Work out the finished part from the listing and answer in its coordinate system (mm). Face numbers are marked on the shaded views. Coordinates: 2 decimals unless noted, no trailing zeros. Order: outer loops, then holes, each group sorted by start corner. A loop starts at its lowest first (then second) coordinate and runs counter-clockwise, first axis right, second up.
1. The part is cut by section B-B, the plane y = -35. Give the vertices of the cut face in (x, z), then the cut area to 3 significant figures.
2. Flat-ended cylindrical pins translate along their axes: pin 1 Ø3.5 at (x, z) = (-9.5, -24) entering from -Y; pin 2 Ø11 at (x, y) = (-1, -16) entering from +Z; pin 3 Ø5 at (x, y) = (2, -10.5) entering from -Z; pin 4 Ø6 at (x, z) = (14.5, 92.5) entering from +Y. Find the tip coordinate at first contact, or state that the pin passes through.
3. Determine the mould class of the marked faces 1, 2, 3 and 4 for opening direction X: +X half, -X half, draft (parallel to the pull), parting line (faces both ways), or undercut.
4. Find the intervals of material crossed by probe 1 along Z at (x, y) = (-9.5, -3.25); probe 2 along Y at (x, z) = (11, -19); probe 3 along X at (y, z) = (-69, 92), in increasing order.
5. The part is cut by section C-C, the plane x = 18. Give the vertices of the cut face in (y, z).
6. The part is cut by section A-A, the plane z = 90.5. Give the vertices of the cut face in (x, y).
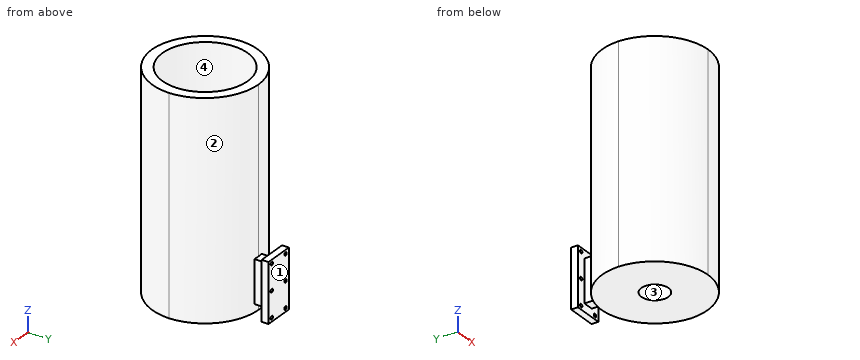
```python
from build123d import *

# Parameters (mm, degrees)
F0_W          = 28
F0_H          = 55
F0_R          = 1.6
F1_DEPTH      = 6.35
F2_W          = 10
F2_H          = 40
F3_DEPTH      = 12.7
F4_W          = 100
F4_H          = 200
F5_DEPTH      = 100
F6_R          = 40
F7_DEPTH      = 177.8
F8_R          = 12.7
F9_DEPTH      = 41.656
F10_T1_DEPTH  = 454
F10_T6_DEPTH  = 454
F10_T12_DEPTH = 454
F10_T18_DEPTH = 454
F10_T25_DEPTH = 454
F10_T31_DEPTH = 454
F10_T37_DEPTH = 454
F10_T43_DEPTH = 454
F10_T49_DEPTH = 454
F10_T56_DEPTH = 454
F10_T62_DEPTH = 454


# Not quite as in the source:
# - a fillet or chamfer that OpenCascade refuses, or shapes differently, is made with other operations: its cross-section is extruded or revolved along the edge and cut away or added


with BuildPart() as f1:
    # F0 (on Front) → F1 (new body)
    with BuildSketch(Plane.XZ):
        Rectangle(F0_W, F0_H)
        with Locations((-9.5, -24)):
            Circle(F0_R, mode=Mode.SUBTRACT)
        with Locations((9.5, -24)):
            Circle(F0_R, mode=Mode.SUBTRACT)
        with Locations((-9.5, 0)):
            Circle(F0_R, mode=Mode.SUBTRACT)
        with Locations((-9.5, 24)):
            Circle(F0_R, mode=Mode.SUBTRACT)
        with Locations((9.5, 0)):
            Circle(F0_R, mode=Mode.SUBTRACT)
        with Locations((9.5, 24)):
            Circle(F0_R, mode=Mode.SUBTRACT)
    extrude(amount=F1_DEPTH)

    # F2 (on face) → F3 (join)
    with BuildSketch(Plane.XZ.offset(6.35)):
        Rectangle(F2_W, F2_H)
    extrude(amount=F3_DEPTH)

    # F4 (on face) → F5 (join)
    with BuildSketch(Plane.XZ.offset(19.05)):
        with Locations((0, 72.5)):
            Rectangle(F4_W, F4_H)
    extrude(amount=F5_DEPTH)

    # F6 (on face) → F7 (cut)
    with BuildSketch(Plane.XY.offset(172.5)):
        with Locations((0, -69.05)):
            Circle(F6_R)
    extrude(amount=-F7_DEPTH, mode=Mode.SUBTRACT)

    # F8 (on face) → F9 (cut)
    with BuildSketch(Plane.XY.offset(-5.3)):
        with Locations((0, -69.05)):
            Circle(F8_R)
    extrude(amount=-F9_DEPTH, mode=Mode.SUBTRACT)

    # F10: fillet of radius 50.8 on 4 edges, made by hand

    # F10_s2 → F10_t1 (cut)
    with BuildSketch(Plane.XY.offset(-154.5)):
        with BuildLine():
            ThreePointArc((-0.8, -119.05), (35.1210244843, -104.1710244843), (50, -68.25))
            Line((50, -68.25), (50, -119.05))
            Line((50, -119.05), (-0.8, -119.05))
        make_face()
        with BuildLine():
            ThreePointArc((-50, -68.25), (-35.1210244843, -104.1710244843), (0.8, -119.05))
            Line((0.8, -119.05), (-50, -119.05))
            Line((-50, -119.05), (-50, -68.25))
        make_face()
    extrude(amount=F10_T1_DEPTH, mode=Mode.SUBTRACT)


with BuildPart() as f10_tool4:
    # F10_s5 → F10_t6 (new body)
    with BuildSketch(Plane.XY.offset(-154.5)):
        with BuildLine():
            ThreePointArc((-0.8, -19.05), (35.1210244843, -33.9289755157), (50, -69.85))
            Line((50, -69.85), (50, -19.05))
            Line((50, -19.05), (-0.8, -19.05))
        make_face()
    extrude(amount=F10_T6_DEPTH)

    split(bisect_by=Plane.XY.offset(-20), keep=Keep.BOTTOM)

    split(bisect_by=Plane.YZ.offset(5), keep=Keep.BOTTOM)


with BuildPart() as f1_1:
    add(f1.part)

    # F10_t3: cut F10_tool4
    add(f10_tool4.part, mode=Mode.SUBTRACT)


with BuildPart() as f10_tool10:
    # F10_s11 → F10_t12 (new body)
    with BuildSketch(Plane.XY.offset(-154.5)):
        with BuildLine():
            ThreePointArc((-0.8, -19.05), (35.1210244843, -33.9289755157), (50, -69.85))
            Line((50, -69.85), (50, -19.05))
            Line((50, -19.05), (-0.8, -19.05))
        make_face()
    extrude(amount=F10_T12_DEPTH)

    split(bisect_by=Plane.XY.offset(-20), keep=Keep.BOTTOM)

    split(bisect_by=Plane.YZ.offset(5), keep=Keep.TOP)


with BuildPart() as f1_2:
    add(f1_1.part)

    # F10_t9: cut F10_tool10
    add(f10_tool10.part, mode=Mode.SUBTRACT)


with BuildPart() as f10_tool16:
    # F10_s17 → F10_t18 (new body)
    with BuildSketch(Plane.XY.offset(-154.5)):
        with BuildLine():
            ThreePointArc((-0.8, -19.05), (35.1210244843, -33.9289755157), (50, -69.85))
            Line((50, -69.85), (50, -19.05))
            Line((50, -19.05), (-0.8, -19.05))
        make_face()
    extrude(amount=F10_T18_DEPTH)

    split(bisect_by=Plane.XY.offset(20), keep=Keep.BOTTOM)

    split(bisect_by=Plane.XY.offset(-20), keep=Keep.TOP)

    split(bisect_by=Plane.YZ.offset(5), keep=Keep.TOP)


with BuildPart() as f1_3:
    add(f1_2.part)

    # F10_t15: cut F10_tool16
    add(f10_tool16.part, mode=Mode.SUBTRACT)


with BuildPart() as f10_tool23:
    # F10_s24 → F10_t25 (new body)
    with BuildSketch(Plane.XY.offset(-154.5)):
        with BuildLine():
            ThreePointArc((-0.8, -19.05), (35.1210244843, -33.9289755157), (50, -69.85))
            Line((50, -69.85), (50, -19.05))
            Line((50, -19.05), (-0.8, -19.05))
        make_face()
    extrude(amount=F10_T25_DEPTH)

    split(bisect_by=Plane.XY.offset(20), keep=Keep.TOP)

    split(bisect_by=Plane.YZ.offset(5), keep=Keep.BOTTOM)


with BuildPart() as f1_4:
    add(f1_3.part)

    # F10_t22: cut F10_tool23
    add(f10_tool23.part, mode=Mode.SUBTRACT)


with BuildPart() as f10_tool29:
    # F10_s30 → F10_t31 (new body)
    with BuildSketch(Plane.XY.offset(-154.5)):
        with BuildLine():
            ThreePointArc((-0.8, -19.05), (35.1210244843, -33.9289755157), (50, -69.85))
            Line((50, -69.85), (50, -19.05))
            Line((50, -19.05), (-0.8, -19.05))
        make_face()
    extrude(amount=F10_T31_DEPTH)

    split(bisect_by=Plane.XY.offset(20), keep=Keep.TOP)

    split(bisect_by=Plane.YZ.offset(5), keep=Keep.TOP)


with BuildPart() as f1_5:
    add(f1_4.part)

    # F10_t28: cut F10_tool29
    add(f10_tool29.part, mode=Mode.SUBTRACT)


with BuildPart() as f10_tool35:
    # F10_s36 → F10_t37 (new body)
    with BuildSketch(Plane.XY.offset(299.5)):
        with BuildLine():
            ThreePointArc((-50, -69.85), (-35.1210244843, -33.9289755157), (0.8, -19.05))
            Line((0.8, -19.05), (-50, -19.05))
            Line((-50, -19.05), (-50, -69.85))
        make_face()
    extrude(amount=-F10_T37_DEPTH)

    split(bisect_by=Plane.XY.offset(20), keep=Keep.TOP)

    split(bisect_by=Plane.YZ.offset(-5), keep=Keep.BOTTOM)


with BuildPart() as f1_6:
    add(f1_5.part)

    # F10_t34: cut F10_tool35
    add(f10_tool35.part, mode=Mode.SUBTRACT)


with BuildPart() as f10_tool41:
    # F10_s42 → F10_t43 (new body)
    with BuildSketch(Plane.XY.offset(299.5)):
        with BuildLine():
            ThreePointArc((-50, -69.85), (-35.1210244843, -33.9289755157), (0.8, -19.05))
            Line((0.8, -19.05), (-50, -19.05))
            Line((-50, -19.05), (-50, -69.85))
        make_face()
    extrude(amount=-F10_T43_DEPTH)

    split(bisect_by=Plane.XY.offset(20), keep=Keep.TOP)

    split(bisect_by=Plane.YZ.offset(-5), keep=Keep.TOP)


with BuildPart() as f1_7:
    add(f1_6.part)

    # F10_t40: cut F10_tool41
    add(f10_tool41.part, mode=Mode.SUBTRACT)


with BuildPart() as f10_tool47:
    # F10_s48 → F10_t49 (new body)
    with BuildSketch(Plane.XY.offset(299.5)):
        with BuildLine():
            ThreePointArc((-50, -69.85), (-35.1210244843, -33.9289755157), (0.8, -19.05))
            Line((0.8, -19.05), (-50, -19.05))
            Line((-50, -19.05), (-50, -69.85))
        make_face()
    extrude(amount=-F10_T49_DEPTH)

    split(bisect_by=Plane.XY.offset(20), keep=Keep.BOTTOM)

    split(bisect_by=Plane.YZ.offset(-5), keep=Keep.BOTTOM)

    split(bisect_by=Plane.XY.offset(-20), keep=Keep.TOP)


with BuildPart() as f1_8:
    add(f1_7.part)

    # F10_t46: cut F10_tool47
    add(f10_tool47.part, mode=Mode.SUBTRACT)


with BuildPart() as f10_tool54:
    # F10_s55 → F10_t56 (new body)
    with BuildSketch(Plane.XY.offset(299.5)):
        with BuildLine():
            ThreePointArc((-50, -69.85), (-35.1210244843, -33.9289755157), (0.8, -19.05))
            Line((0.8, -19.05), (-50, -19.05))
            Line((-50, -19.05), (-50, -69.85))
        make_face()
    extrude(amount=-F10_T56_DEPTH)

    split(bisect_by=Plane.YZ.offset(-5), keep=Keep.BOTTOM)

    split(bisect_by=Plane.XY.offset(-20), keep=Keep.BOTTOM)


with BuildPart() as f1_9:
    add(f1_8.part)

    # F10_t53: cut F10_tool54
    add(f10_tool54.part, mode=Mode.SUBTRACT)


with BuildPart() as f10_tool60:
    # F10_s61 → F10_t62 (new body)
    with BuildSketch(Plane.XY.offset(299.5)):
        with BuildLine():
            ThreePointArc((-50, -69.85), (-35.1210244843, -33.9289755157), (0.8, -19.05))
            Line((0.8, -19.05), (-50, -19.05))
            Line((-50, -19.05), (-50, -69.85))
        make_face()
    extrude(amount=-F10_T62_DEPTH)

    split(bisect_by=Plane.YZ.offset(-5), keep=Keep.TOP)

    split(bisect_by=Plane.XY.offset(-20), keep=Keep.BOTTOM)


with BuildPart() as f1_10:
    add(f1_9.part)

    # F10_t59: cut F10_tool60
    add(f10_tool60.part, mode=Mode.SUBTRACT)


solid = f1_10.part
```
Geometry says:
1. outline: (-36.16, -27.5) - (36.16, -27.5) - (36.16, 172.5) - (20.99, 172.5) - (20.99, -5.3) - (-20.99, -5.3) - (-20.99, 172.5) - (-36.16, 172.5) - close
1. area: 7,000 mm2
2. pin 1: stops at y = -118.33
2. pin 2: stops at z = 172.5
2. pin 3: stops at z = -20
2. pin 4: stops at y = -20.56
3. face 1: draft
3. face 2: +X half
3. face 3: undercut
3. face 4: undercut
4. probe 1: z = -27.5 to -25.6, -22.4 to -1.6, 1.6 to 22.4, 25.6 to 27.5
4. probe 2: y = -117.66 to -75.4, -62.7 to -20.44, -6.35 to 0
4. probe 3: x = -49.99 to -40, 40 to 49.99
5. outline: (-115.44, -27.5) - (-22.66, -27.5) - (-22.66, 172.5) - (-33.33, 172.5) - (-33.33, -5.3) - (-104.77, -5.3) - (-104.77, 172.5) - (-115.44, 172.5) - close
6. outline: (-49.99, -69.05) arc R50.8 ccw to (0, -119.04) arc R50.8 ccw to (49.99, -69.05) arc R50.8 ccw to (0, -19.06) arc R50.8 ccw to start; hole circle Ø80 at (0, -69.05)
